Geometry: final body of the model. Coordinates: model frame, mm. A direction names the side the tool comes from. Give positions to 0.01 mm unless a question says otherwise; leave off trailing zeros. Write each loop counter-clockwise with the first axis right and the second up, starting at its lowest first coordinate (ties: lowest second). Pieces come first, ordered by that corner, then holes.
Q1. Cut plane B-B on y = 24.5. Return the cut outline in (x, z), plus the area to 3 significant figures.
Q2. Draft query along Y for faces 1 (the face through (-2, 45, -104)), 2 (the face through (-2, 0, -66)), 3 (the face through (-2, 2, -72)). Return one class per face: pulls with the +Y half, pulls with the -Y half, needs draft (parallel to the pull), parting line crosses it, or undercut.
Q3. Cut plane A-A on x = -1.2. Count the separate pieces of the cut face and the enclosed holes in it, plus the area to 3 significant figures.
Q4. Reachability of faces 4 (the face through (-2, 8, -4)), 5 (the face through (-2, 2, -96)), 6 (the face through (-2, 21, -106)) from +Z, -Z, +X, -X, +Y, -Y: full face, straight path, thin tool, end or side. Return the list, or none.
Q5. Cut plane C-C on z = -78.5. Return the cut outline in (x, y), plus the area to 3 significant figures.
Q6. Pin query (flat end, axial travel): pin 1 (1.5 mm diameter, centred on x = -3, y = 26.5, fed in from +Z); pin 2 (1.2 mm diameter, centred on x = -3, z = -2, fed in from +Y); pin 3 (1.2 mm diameter, centred on x = -2, y = 7.5, fed in from -Z); pin 4 (10 mm diameter, centred on y = 19, z = -28, fed in from +X). Return the tip coordinate at first contact, or that it passes through.
Q7. Line query: L1, parallel to Z at x = -0.85, y = 43; L2, parallel to Y at x = -3.6, z = -67; L3, parallel to Y at x = -1.2, z = -32. Output: solid intervals per line, ascending.
Autodesk Inventor part; units mm, degrees
ref_plane "YZ Plane" through (0, 0, 0) normal (1, 0, 0) x (0, 1, 0)
ref_plane "XZ Plane" through (0, 0, 0) normal (0, 1, 0) x (-1, 0, 0)
ref_plane "XY Plane" through (0, 0, 0) normal (0, 0, 1) x (1, 0, 0)
sketch "Sketch1" plane through (0, 0, 0) normal (1, 0, 0) x (0, 1, 0)
  line L0 (0, 0) -> (69, 0)
  line L1 (69, 0) -> (69, -108)
  line L2 (69, -108) -> (0, -108)
  line L3 (0, -108) -> (0, 0)
  dimension "d228" = 69
  dimension "d229" = 108
extrude "Extrusion1" add sketch "Sketch1" against normal blind 4
sketch "Sketch2" plane through (0, 0, 0) normal (1, 0, 0) x (0, 0, -1)
  line L0 (54, 69) -> (54, 0)
  line L1 (108, 0) -> (0, 0)
  line L2 (0, 0) -> (0, 69)
  line L3 (0, 34.5) -> (108, 34.5)
  line L4 (108, 69) -> (108, 0)
  line L5 (0, 0) -> (108, 0)
  line L6 (12, 0) -> (12, 4)
  line L7 (4, 0) -> (12, 0)
  line L8 (4, 59) -> (4, 49)
  line L9 (4, 49) -> (0, 49)
  line L10 (0, 49) -> (0, 41)
  line L11 (0, 41) -> (4, 41)
  line L12 (4, 41) -> (4, 29)
  line L13 (4, 29) -> (0, 29)
  line L14 (0, 29) -> (0, 21)
  line L15 (0, 21) -> (4, 21)
  line L16 (4, 21) -> (4, 11)
  line L17 (4, 11) -> (0, 11)
  line L18 (0, 69) -> (0, 0)
  line L19 (108, 0) -> (108, 69)
  line L20 (108, 34.5) -> (0, 34.5)
  line L21 (108, 49) -> (108, 41)
  line L22 (108, 29) -> (108, 21)
  line L23 (108, 69) -> (108, 0)
  line L24 (4, 59) -> (0, 59)
  line L25 (0, 0) -> (108, 0)
  line L26 (108, 69) -> (0, 69)
  line L27 (108, 0) -> (108, 69)
  line L28 (108, 34.5) -> (0, 34.5)
  line L29 (104, 59) -> (104, 49)
  line L30 (104, 49) -> (108, 49)
  line L31 (108, 49) -> (108, 41)
  line L32 (108, 41) -> (104, 41)
  line L33 (104, 41) -> (104, 29)
  line L34 (104, 29) -> (108, 29)
  line L35 (108, 29) -> (108, 21)
  line L36 (108, 21) -> (104, 21)
  line L37 (104, 21) -> (104, 11)
  line L38 (104, 11) -> (108, 11)
  line L39 (108, 69) -> (108, 0)
  line L40 (0, 34.5) -> (108, 34.5)
  line L41 (104, 59) -> (108, 59)
  line L42 (4, 49) -> (4, 41)
  line L43 (4, 29) -> (4, 21)
  line L44 (4, 59) -> (4, 69)
  line L45 (0, 69) -> (108, 69)
  line L46 (104, 69) -> (104, 59)
  line L47 (104, 49) -> (104, 41)
  line L48 (104, 29) -> (104, 21)
  line L49 (12, 0) -> (24, 0)
  line L50 (24, 0) -> (24, 4)
  line L51 (24, 4) -> (36, 4)
  line L52 (36, 4) -> (36, 0)
  line L53 (36, 0) -> (24, 0)
  line L54 (36, 0) -> (48, 0)
  line L55 (60, 0) -> (48, 0)
  line L56 (60, 0) -> (72, 0)
  line L57 (72, 0) -> (72, 4)
  line L58 (72, 4) -> (84, 4)
  line L59 (84, 4) -> (84, 0)
  line L60 (84, 0) -> (72, 0)
  line L61 (12, 4) -> (0, 4)
  line L62 (4, 11) -> (4, 0)
  line L63 (104, 11) -> (104, 0)
  line L64 (106, 0) -> (96, 0)
  line L65 (84, 0) -> (96, 0)
  line L66 (48, 0) -> (60, 0)
  line L67 (60, 0) -> (72, 0)
  line L68 (96, 0) -> (106, 0)
  line L69 (108, 4) -> (108, 11)
  line L70 (60, 0) -> (60, 4)
  line L71 (48, 4) -> (48, 0)
  line L72 (60, 4) -> (48, 4)
  line L73 (96, 4) -> (108, 4)
  line L74 (96, 4) -> (96, 0)
  line L75 (108, 0) -> (108, 69)
  line L76 (108, 4) -> (108, 0)
  point P0 (12, 0)
  point P1 (108, 29)
  point P2 (108, 41)
  point P3 (108, 49)
  point P4 (108, 59)
  point P5 (108, 11)
  point P6 (108, 21)
  point P7 (84, 0)
  point P8 (104, 0)
  point P9 (36, 0)
  point P10 (4, 4)
  point P11 (104, 4)
  dimension "d246" = 12
  dimension "d248" = 10
  dimension "d250" = 8
  dimension "d253" = 4
  dimension "d256" = 10
  dimension "d257" = 12
  dimension "d259" = 12
extrude "Extrusion2" cut sketch "Sketch2" against normal blind 4 contours L26 L4 L41 L46 | L44 L24 L2 L26 | L72 L70 L1 L0 | L0 L1 L71 L72 | L11 L2 L9 L42 | L43 L15 L2 L13 | L47 L30 L4 L32 | L34 L4 L36 L48 | L57 L58 L59 L1 | L1 L50 L51 L52 | L62 L61 L2 L17 | L38 L4 L73 L63 | L62 L1 L2 L61 | L61 L6 L1 L62 | L73 L4 L1 L63 | L63 L1 L74 L73
sketch "Sketch3" plane through (0, 0, 0) normal (1, 0, 0) x (0, 0, -1)
  line L0 (41, 39.5) -> (81, 39.5)
  line L1 (81, 39.5) -> (81, 43.5)
  line L2 (81, 43.5) -> (41, 43.5)
  line L3 (41, 43.5) -> (41, 39.5)
  line L4 (48, 4) -> (60, 4)
  line L5 (67, 43.5) -> (67, 39.5)
  line L6 (104, 69) -> (4, 69)
  line L7 (54, 69) -> (54, 4)
  line L8 (60, 4) -> (48, 4)
  line L9 (51, 43.5) -> (51, 39.5)
  line L10 (81, 43.5) -> (91, 43.5)
  line L11 (91, 43.5) -> (91, 39.5)
  line L12 (91, 39.5) -> (81, 39.5)
  line L13 (81, 39.5) -> (81, 43.5)
  line L14 (61, 43.5) -> (61, 39.5)
  line L15 (71, 43.5) -> (71, 39.5)
  point P0 (0, 0)
  dimension "d265" = 35.5
  dimension "d266" = 26
  dimension "d267" = 10
  dimension "d272" = 4
  dimension "d274" = 10
  dimension "d275" = 10
  dimension "d276" = 10
  dimension "d277" = 10
extrude "Extrusion3" cut sketch "Sketch3" against normal blind 4 contours L3 L2 L9 L0 | L14 L2 L5 L0 | L5 L2 L15 L0 | L1 L10 L11 L12
properties part number "Langbektang houder"
Data:
1. outline: (-4, -104) - (0, -104) - (0, -4) - (-4, -4) - close
1. area: 400 mm2
2. face 1: undercut
2. face 2: pulls with the -Y half
2. face 3: needs draft
3. separate pieces: 1
3. enclosed holes: 3
3. area: 6,830 mm2
4. face 4: +Z, +X, -X, -Y
4. face 5: -Z, +X, -X, -Y
4. face 6: -Z, +X, -X
5. outline: (-4, 4) - (0, 4) - (0, 69) - (-4, 69) - close
5. area: 260 mm2
6. pin 1: stops at z = -4
6. pin 2: stops at y = 59
6. pin 3: stops at z = -104
6. pin 4: stops at x = 0
7. L1: z = -104 to -91, -81 to -71, -61 to -51, -41 to -4
7. L2: y = 0 to 39.5, 43.5 to 69
7. L3: y = 4 to 69
